Autodesk Inventor part; units mm, degrees
ref_plane "socket_to_dummy_XY" through (0, 0, 0) normal (0, -1, 0) x (1, 0, 0)
ref_plane "socket_to_dummy_YZ" through (0, 0, 0) normal (1, 0, 0) x (0, 0, 1)
ref_plane "socket_to_dummy_ZX" through (0, 0, 0) normal (0, 0, 1) x (0, -1, 0)
sketch "Sketch_1" plane through (0, 0, 0) normal (0, 1, 0) x (1, 0, 0)
  line L0 (-8.89, 2.54) -> (-8.89, -2.54)
  line L1 (-8.89, -2.54) -> (8.89, -2.54)
  line L2 (8.89, -2.54) -> (8.89, 2.54)
  line L3 (8.89, 2.54) -> (-8.89, 2.54)
  line L4 (7.239, -0.889) -> (7.239, -1.651)
  line L5 (7.239, -1.651) -> (8.001, -1.651)
  line L6 (8.001, -1.651) -> (8.001, -0.889)
  line L7 (8.001, -0.889) -> (7.239, -0.889)
  line L8 (7.239, 1.651) -> (7.239, 0.889)
  line L9 (7.239, 0.889) -> (8.001, 0.889)
  line L10 (8.001, 0.889) -> (8.001, 1.651)
  line L11 (8.001, 1.651) -> (7.239, 1.651)
  line L12 (4.699, -0.889) -> (4.699, -1.651)
  line L13 (4.699, -1.651) -> (5.461, -1.651)
  line L14 (5.461, -1.651) -> (5.461, -0.889)
  line L15 (5.461, -0.889) -> (4.699, -0.889)
  line L16 (4.699, 1.651) -> (4.699, 0.889)
  line L17 (4.699, 0.889) -> (5.461, 0.889)
  line L18 (5.461, 0.889) -> (5.461, 1.651)
  line L19 (5.461, 1.651) -> (4.699, 1.651)
  line L20 (2.159, -0.889) -> (2.159, -1.651)
  line L21 (2.159, -1.651) -> (2.921, -1.651)
  line L22 (2.921, -1.651) -> (2.921, -0.889)
  line L23 (2.921, -0.889) -> (2.159, -0.889)
  line L24 (2.159, 1.651) -> (2.159, 0.889)
  line L25 (2.159, 0.889) -> (2.921, 0.889)
  line L26 (2.921, 0.889) -> (2.921, 1.651)
  line L27 (2.921, 1.651) -> (2.159, 1.651)
  line L28 (-0.381, -0.889) -> (-0.381, -1.651)
  line L29 (-0.381, -1.651) -> (0.381, -1.651)
  line L30 (0.381, -1.651) -> (0.381, -0.889)
  line L31 (0.381, -0.889) -> (-0.381, -0.889)
  line L32 (-0.381, 1.651) -> (-0.381, 0.889)
  line L33 (-0.381, 0.889) -> (0.381, 0.889)
  line L34 (0.381, 0.889) -> (0.381, 1.651)
  line L35 (0.381, 1.651) -> (-0.381, 1.651)
  line L36 (-2.921, -0.889) -> (-2.921, -1.651)
  line L37 (-2.921, -1.651) -> (-2.159, -1.651)
  line L38 (-2.159, -1.651) -> (-2.159, -0.889)
  line L39 (-2.159, -0.889) -> (-2.921, -0.889)
  line L40 (-2.921, 1.651) -> (-2.921, 0.889)
  line L41 (-2.921, 0.889) -> (-2.159, 0.889)
  line L42 (-2.159, 0.889) -> (-2.159, 1.651)
  line L43 (-2.159, 1.651) -> (-2.921, 1.651)
  line L44 (-5.461, -0.889) -> (-5.461, -1.651)
  line L45 (-5.461, -1.651) -> (-4.699, -1.651)
  line L46 (-4.699, -1.651) -> (-4.699, -0.889)
  line L47 (-4.699, -0.889) -> (-5.461, -0.889)
  line L48 (-5.461, 1.651) -> (-5.461, 0.889)
  line L49 (-5.461, 0.889) -> (-4.699, 0.889)
  line L50 (-4.699, 0.889) -> (-4.699, 1.651)
  line L51 (-4.699, 1.651) -> (-5.461, 1.651)
  line L52 (-8.001, -0.889) -> (-8.001, -1.651)
  line L53 (-8.001, -1.651) -> (-7.239, -1.651)
  line L54 (-7.239, -1.651) -> (-7.239, -0.889)
  line L55 (-7.239, -0.889) -> (-8.001, -0.889)
  line L56 (-8.001, 1.651) -> (-8.001, 0.889)
  line L57 (-8.001, 0.889) -> (-7.239, 0.889)
  line L58 (-7.239, 0.889) -> (-7.239, 1.651)
  line L59 (-7.239, 1.651) -> (-8.001, 1.651)
extrude "Extrusion1" add sketch "Sketch_1" along normal blind 3.5052
sketch "Sketch_4" plane through (0, 0, 0) normal (1, 0, 0) x (0, 1, 0)
  line L0 (0.254, 2.032) -> (0, 2.032)
  line L1 (0, 2.032) -> (0, -2.032)
  line L2 (0, -2.032) -> (0.254, -2.032)
  line L3 (0.254, -2.032) -> (0.254, 2.032)
extrude "Extrusion2" cut sketch "Sketch_4" along normal mid plane 17.78
sketch "Sketch_9" plane through (0, 0, 0) normal (0, 0, 1) x (1, 0, 0)
  line L0 (6.35, -1.27) -> (6.35, 0.635)
  line L1 (6.35, 0.635) -> (7.1437, 0.635)
  line L2 (7.1437, 0.635) -> (7.1437, -0.9842)
  arc A0 (6.858, -1.27) -> (7.1437, -0.9842) centre (6.858, -0.9843) ccw
  line L3 (6.858, -1.27) -> (6.35, -1.27)
  line L4 (6.35, -1.27) -> (6.35, 0.635)
revolve "Revolution1" add sketch "Sketch_9" angle 360 about axis through (6.35, -1.27, 0) along (0, -1, 0)
sketch "Sketch_10" plane through (0, 0, 0) normal (0, 0, 1) x (1, 0, 0)
  line L0 (-6.35, -1.27) -> (-6.35, 0.635)
  line L1 (-6.35, 0.635) -> (-5.5563, 0.635)
  line L2 (-5.5563, 0.635) -> (-5.5563, -0.9525)
  arc A0 (-5.8738, -1.27) -> (-5.5563, -0.9525) centre (-5.8738, -0.9525) ccw
  line L3 (-5.8738, -1.27) -> (-6.35, -1.27)
  line L4 (-6.35, -1.27) -> (-6.35, 0.635)
revolve "Revolution2" add sketch "Sketch_10" angle 360 about axis through (-6.35, -1.27, 0) along (0, -1, 0)
sketch "Sketch_11" plane through (0, 3.5052, 0) normal (0, 1, 0) x (1, 0, 0)
  line L0 (-6.5405, 1.27) -> (-6.5405, -1.27)
  line L1 (-6.5405, -1.27) -> (-6.1595, -1.27)
  line L2 (-6.1595, -1.27) -> (-6.1595, 1.27)
  line L3 (-6.1595, 1.27) -> (-6.5405, 1.27)
extrude "Extrusion3" cut sketch "Sketch_11" against normal blind 1.27
pattern_linear "Rectangular Pattern1" count 6 spacing 2.54 along (1, 0, 0) of "Extrusion3"
ref_plane "socket_to_dummy_XY" through (0, 0, 0) normal (0, -1, 0) x (1, 0, 0)
ref_plane "socket_to_dummy_YZ" through (0, 0, 0) normal (1, 0, 0) x (0, 0, 1)
ref_plane "socket_to_dummy_ZX" through (0, 0, 0) normal (0, 0, 1) x (0, -1, 0)
ref_plane "socket_to_pad_XY" through (0, 3.5052, 0) normal (0, 1, 0) x (1, 0, 0)
ref_plane "socket_to_pad_YZ" through (0, 3.5052, 0) normal (1, 0, 0) x (0, 0, -1)
ref_plane "socket_to_pad_ZX" through (0, 3.5052, 0) normal (0, 0, -1) x (0, 1, 0)
properties part number "HLE-107-02-DV-A_socket"
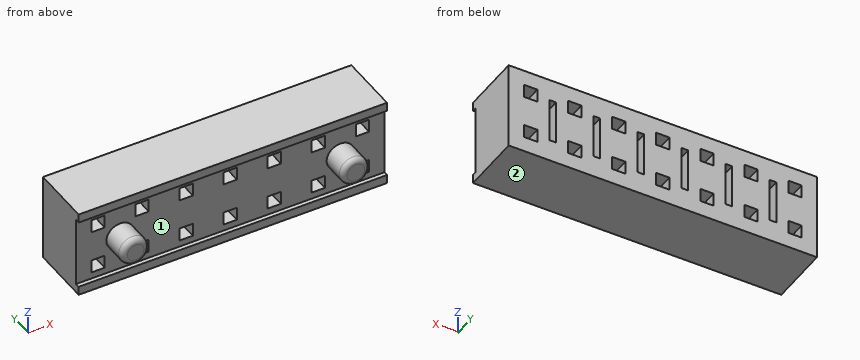
Model file for the job. Use its own axes, mm. Face numbers are marked on the shaded views. A direction names the side the tool comes from. Coordinates: 2 decimals unless noted, no trailing zeros. Loops run counter-clockwise (first coordinate to the right, second up) from the corner with the lowest first, then second, coordinate; pieces in that order, holes last. Notation, with made-up numbers: (46.25, 15.25) - (90.25, 15.25) arc R18 ccw to (90.25, 38.25) - close; hole circle Ø3 at (2.5, 59.25). An arc over 180 degrees is marked (long way). Answer as a JSON object with one key per item and string values. Group by question number.
(1) Tool access for the marked faces 1 and 2: list every direction of +Z, -Z, +X, -X, +Y, -Y with a clear straight run to the whole face (end or side of a thin tool).
(2) Probe line 1 along Z through (x, y) = (-2.25, 3.35); line 2 along Z through (x, y) = (7, 0.05); line 3 along Y through (x, z) = (5.75, 1.45). List the from-to ranges inside material, lowest first.
(3) Cut at A-A (x = 2.5). Give the cut face in (y, z), then the cut area to 3 significant figures.
(4) Cut at B-B (z = 1.1). State how many separate pieces and enclosed holes the cut face has, then the cut area to 3 significant figures.
(5) Cut at D-D (y = -0.35). Give the cut face in (x, z), then the cut area to 3 significant figures.
Geometry says:
{
 "1": {"face 1": "-Y", "face 2": "-Z, +X, -X, +Y, -Y"},
 "2": {"line 1": "z = -2.54 to -1.65, -0.89 to 0.89, 1.65 to 2.54", "line 2": "z = -2.54 to -2.03, -0.46 to 0.46, 2.03 to 2.54", "line 3": "y = 0.25 to 3.51"},
 "3": {"outline": "(0, -2.54) - (3.51, -2.54) - (3.51, -1.65) - (0.25, -1.65) - (0.25, -2.03) - (0, -2.03) - close; (0, 2.03) - (0.25, 2.03) - (0.25, 1.65) - (3.51, 1.65) - (3.51, 2.54) - (0, 2.54) - close; (0.25, -0.89) - (3.51, -0.89) - (3.51, 0.89) - (0.25, 0.89) - close", "area": "11.8 mm^2"},
 "4": {"separate pieces": "8", "enclosed holes": "0", "area": "37.6 mm^2"},
 "5": {"outline": "circle Ø1.59 at (-6.35, 0); circle Ø1.59 at (6.35, 0)", "area": "3.96 mm^2"}
}
